Design review of the part built by this model. Coordinates are the model's own, in mm. A direction names the side the tool comes from. Coordinates: 2 decimals unless noted, no trailing zeros. Write each loop counter-clockwise with the first axis right and the second up, starting at its lowest first coordinate (ties: lowest second). Pieces come first, ordered by that corner, then holes.
Q1. Mouldability with a two-part tool opening along X and no side actions: class faces 4 (the cylindrical face through (-33.416, 29.257, 43.021)), 5 (the flat face through (35.84, 42.41, 0.21)), 6 (the cylindrical face through (4.38, -8.43, 47.54)), 7 (the flat face through (-7, -35.5, 1)) as pulls with the +X half, pulls with the -X half, needs draft (parallel to the pull), parting line crosses it, or undercut.
Q2. Take a section at A-A (z = 1.5). Give the boundary of the cut face in (x, y).
Q3. Take a section at B-B (z = -37.5). Give the boundary of the cut face in (x, y).
Q4. Machinability: for faces 1 (the flat face through (-34.09, -15.44, -42.98)), 2 (the flat face through (-33.94, 15.06, -42.98)), 3 (the flat face through (29, 40, 15)), which of the approach directions +Z, -Z, +X, -X, +Y, -Y give a long, thin tool a straight path to every point of the face, cutting with its end or side? Answer none if there is none.
Q5. Take a section at C-C (y = -16). Give the boundary of the cut face in (x, z), and give its area (3 significant figures).
Q6. For probe 1 along Y at (x, z) = (28, -1.75); probe 2 along X at (y, z) = (7.5, -36.5); probe 3 along Z at (x, y) = (-31.5, -30.5), list the stretches that pass through material, from the lowest coordinate up.
Q7. Take a section at D-D (x = 4.5). Give the boundary of the cut face in (y, z).
Q8. Insertion check: pin 1 (8 mm diameter, centred on y = 6, z = -27, fed in from +X); pin 2 (6 mm diameter, centred on x = -29.5, z = -9, fed in from -Y); pin 3 (8 mm diameter, centred on x = -34, y = 37, fed in from +Z); pin 4 (3 mm diameter, centred on x = -31.5, y = 27.5, fed in from -Z). Each pin has a flat end and moves straight along its axis. Give the tip position at first contact, or say it passes through.
```python
from build123d import *

# Parameters (mm, degrees)
SKETCH_1_W          = 46
SKETCH_1_H          = 89
EXTRUDE_1_DEPTH     = 35.5
SKETCH_3_R          = 2.6
EXTRUDE_2_DEPTH     = 3
EXTRUDE_START       = -3
SKETCH_4_R          = 2.6
EXTRUDE_3_DEPTH     = 3
SKETCH_5_R          = 14
EXTRUDE_4_DEPTH     = 6
SKETCH_6_R          = 11.5
CUT_EXTRUDE_1_DEPTH = 88.954242748
SKETCH_7_R          = 2.6
EXTRUDE_5_DEPTH     = 15
SKETCH_8_R          = 1.9
SKETCH_8_R_2        = 4.5
EXTRUDE_6_DEPTH     = 15
SKETCH_9_R          = 2.6
CUT_EXTRUDE_2_DEPTH = 115.249255194
SKETCH_10_R         = 9.5
CUT_EXTRUDE_3_DEPTH = 6
SKETCH_11_R         = 7.5
CUT_EXTRUDE_4_DEPTH = 6
SKETCH_12_R         = 9.5
CUT_EXTRUDE_5_DEPTH = 6


with BuildPart() as part:
    # 草图1 → 凸台-拉伸1 (new, symmetric)
    with BuildSketch(Plane(origin=(0, 0, 0), x_dir=(1, 0, 0), z_dir=(0, 1, 0))):
        Rectangle(SKETCH_1_W, SKETCH_1_H)
    extrude(amount=EXTRUDE_1_DEPTH, both=True)

    # 草图3 → 凸台-拉伸2 (add)
    # profile 1 of 2: a face of its own
    with BuildSketch(Plane.XY.offset(44.5)):
        with BuildLine():
            Line((23, 35.5), (34.653402281, 35.5))
            ThreePointArc((34.653402281, 35.5), (38.786905937, 33.313209471), (39.304766934, 28.66565901))
            Line((39.304766934, 28.66565901), (28.72340208, 1.83434099))
            ThreePointArc((28.72340208, 1.83434099), (28.374766733, 0), (28.72340208, -1.83434099))
            Line((28.72340208, -1.83434099), (39.304766934, -28.66565901))
            ThreePointArc((39.304766934, -28.66565901), (38.786905937, -33.313209471), (34.653402281, -35.5))
            Line((34.653402281, -35.5), (23, -35.5))
            Line((23, -35.5), (23, 35.5))
        make_face()
        with Locations((31.5, 27.5)):
            Circle(SKETCH_3_R, mode=Mode.SUBTRACT)
        with Locations((31.5, -27.5)):
            Circle(SKETCH_3_R, mode=Mode.SUBTRACT)
    # profile 2 of 2: a face of its own
    with BuildSketch(Plane.XY.offset(44.5)):
        with BuildLine():
            Line((-23, -35.5), (-23, 35.5))
            Line((-23, 35.5), (-34.653402281, 35.5))
            ThreePointArc((-34.653402281, 35.5), (-38.786905937, 33.313209471), (-39.304766934, 28.66565901))
            Line((-39.304766934, 28.66565901), (-28.72340208, 1.83434099))
            ThreePointArc((-28.72340208, 1.83434099), (-28.374766733, 0), (-28.72340208, -1.83434099))
            Line((-28.72340208, -1.83434099), (-39.304766934, -28.66565901))
            ThreePointArc((-39.304766934, -28.66565901), (-38.786905937, -33.313209471), (-34.653402281, -35.5))
            Line((-34.653402281, -35.5), (-23, -35.5))
        make_face()
        with Locations((-31.5, -27.5)):
            Circle(SKETCH_3_R, mode=Mode.SUBTRACT)
        with Locations((-31.5, 27.5)):
            Circle(SKETCH_3_R, mode=Mode.SUBTRACT)
    extrude(amount=-EXTRUDE_2_DEPTH)

    # 草图4 → 凸台-拉伸3 (add)
    # profile 1 of 2: a face of its own
    with BuildSketch(Plane(origin=(0, 0, -44.5), x_dir=(-1, 0, 0), z_dir=(0, 0, -1)).offset(EXTRUDE_START)):
        with BuildLine():
            Line((39.304766934, -28.66565901), (28.72340208, -1.83434099))
            ThreePointArc((28.72340208, -1.83434099), (28.374766733, 0), (28.72340208, 1.83434099))
            Line((28.72340208, 1.83434099), (39.304766934, 28.66565901))
            ThreePointArc((39.304766934, 28.66565901), (38.786905937, 33.313209471), (34.653402281, 35.5))
            Line((34.653402281, 35.5), (23, 35.5))
            Line((23, 35.5), (23, -35.5))
            Line((23, -35.5), (34.653402281, -35.5))
            ThreePointArc((34.653402281, -35.5), (38.786905937, -33.313209471), (39.304766934, -28.66565901))
        make_face()
        with Locations(Location((31.5, 27.5, 0), (0, 0, 180))):
            Circle(SKETCH_4_R, mode=Mode.SUBTRACT)
        with Locations(Location((31.5, -27.5, 0), (0, 0, 180))):
            Circle(SKETCH_4_R, mode=Mode.SUBTRACT)
    # profile 2 of 2: a face of its own
    with BuildSketch(Plane(origin=(0, 0, -44.5), x_dir=(-1, 0, 0), z_dir=(0, 0, -1)).offset(EXTRUDE_START)):
        with BuildLine():
            Line((-23, 35.5), (-34.653402281, 35.5))
            ThreePointArc((-34.653402281, 35.5), (-38.786905937, 33.313209471), (-39.304766934, 28.66565901))
            Line((-39.304766934, 28.66565901), (-28.72340208, 1.83434099))
            ThreePointArc((-28.72340208, 1.83434099), (-28.374766733, 0), (-28.72340208, -1.83434099))
            Line((-28.72340208, -1.83434099), (-39.304766934, -28.66565901))
            ThreePointArc((-39.304766934, -28.66565901), (-38.786905937, -33.313209471), (-34.653402281, -35.5))
            Line((-34.653402281, -35.5), (-23, -35.5))
            Line((-23, -35.5), (-23, 35.5))
        make_face()
        with Locations(Location((-31.5, -27.5, 0), (0, 0, 180))):
            Circle(SKETCH_4_R, mode=Mode.SUBTRACT)
        with Locations(Location((-31.5, 27.5, 0), (0, 0, 180))):
            Circle(SKETCH_4_R, mode=Mode.SUBTRACT)
    extrude(amount=EXTRUDE_3_DEPTH)

    # 草图5 → 凸台-拉伸4 (add)
    with BuildSketch(Plane.XY.offset(44.5)):
        Circle(SKETCH_5_R)
    extrude(amount=EXTRUDE_4_DEPTH)

    # 草图6 → 切除-拉伸1 (cut, through all)
    with BuildSketch(Plane(origin=(23, 0, 0), x_dir=(0, 0, -1), z_dir=(1, 0, 0))):
        with Locations((-1.5, 0)):
            Circle(SKETCH_6_R)
    extrude(amount=-CUT_EXTRUDE_1_DEPTH, mode=Mode.SUBTRACT)

    # 草图7 → 凸台-拉伸5 (add, symmetric)
    with BuildSketch(Plane.XY):
        with BuildLine():
            Line((23, 19.5), (23, 35.5))
            Line((23, 35.5), (31.5, 35.5))
            ThreePointArc((31.5, 35.5), (39.5, 27.5), (31.5, 19.5))
            Line((31.5, 19.5), (23, 19.5))
        make_face()
        with Locations((31.5, 27.5)):
            Circle(SKETCH_7_R, mode=Mode.SUBTRACT)
    extrude_5 = extrude(amount=EXTRUDE_5_DEPTH, both=True)

    # 镜向1: 凸台-拉伸5 across plane
    add(extrude_5.mirror(Plane(origin=(0, 0, 0), x_dir=(0, 0, 1), z_dir=(1, 0, 0))))

    # 草图8 → 凸台-拉伸6 (add, symmetric)
    # profile 1 of 2: a face of its own
    with BuildSketch(Plane.XY):
        with BuildLine():
            Line((39.235581788, 29.539797639), (32.351264755, 55.647386172))
            ThreePointArc((32.351264755, 55.647386172), (32.46266128, 55.078493129), (32.5, 54.5))
            ThreePointArc((32.5, 54.5), (28, 50), (23.5, 54.5))
            Line((23.5, 54.5), (23.5, 35.5))
            Line((23.5, 35.5), (31.5, 35.5))
            ThreePointArc((31.5, 35.5), (36.382705136, 33.837127942), (39.235581788, 29.539797639))
        make_face()
        with Locations((28, 42.5)):
            Circle(SKETCH_8_R, mode=Mode.SUBTRACT)
    # profile 2 of 2: a face of its own
    with BuildSketch(Plane.XY):
        with Locations((28, 54.5)):
            Circle(SKETCH_8_R_2)
        with Locations((28, 54.5)):
            Circle(SKETCH_8_R, mode=Mode.SUBTRACT)
    extrude_6 = extrude(amount=EXTRUDE_6_DEPTH, both=True)

    # 镜向2: 凸台-拉伸5, 凸台-拉伸6 across plane
    add(extrude_5.mirror(Plane(origin=(0, 0, 0), x_dir=(0, 0, 1), z_dir=(1, 0, 0))))
    add(extrude_6.mirror(Plane(origin=(0, 0, 0), x_dir=(0, 0, 1), z_dir=(1, 0, 0))))

    # 草图9 → 切除-拉伸2 (cut, through all)
    with BuildSketch(Plane.XZ.offset(35.5)):
        with Locations(Location((15, -37.5, 0), (0, 0, 270))):
            Circle(SKETCH_9_R)
        with Locations(Location((-15, -37.5, 0), (0, 0, 270))):
            Circle(SKETCH_9_R)
        with Locations(Location((-15, 37.5, 0), (0, 0, 270))):
            Circle(SKETCH_9_R)
        with Locations(Location((15, 37.5, 0), (0, 0, 270))):
            Circle(SKETCH_9_R)
    extrude(amount=-CUT_EXTRUDE_2_DEPTH, mode=Mode.SUBTRACT)

    # 草图10 → 切除-拉伸3 (cut)
    with BuildSketch(Plane.XY.offset(50.5)):
        Circle(SKETCH_10_R)
    extrude(amount=-CUT_EXTRUDE_3_DEPTH, mode=Mode.SUBTRACT)

    # 草图11 → 切除-拉伸4 (cut)
    with BuildSketch(Plane.XY.offset(44.5)):
        Circle(SKETCH_11_R)
    extrude(amount=-CUT_EXTRUDE_4_DEPTH, mode=Mode.SUBTRACT)

    # 草图12 → 切除-拉伸5 (cut)
    with BuildSketch(Plane.XY.offset(38.5)):
        Circle(SKETCH_12_R)
    extrude(amount=-CUT_EXTRUDE_5_DEPTH, mode=Mode.SUBTRACT)


solid = part.part
```
Response:
1. face 4: undercut
1. face 5: pulls with the +X half
1. face 6: undercut
1. face 7: needs draft
2. outline: (-39.24, 29.54) arc R8 ccw to (-31.5, 19.5) - (-23, 19.5) - (-23, 11.5) - (23, 11.5) - (23, 19.5) - (31.5, 19.5) arc R8 ccw to (39.24, 29.54) - (32.35, 55.65) arc R4.5 ccw to (23.5, 54.5) - (23.5, 35.5) - (-23.5, 35.5) - (-23.5, 54.5) arc R4.5 ccw to (-32.35, 55.65) - close; (-23, -35.5) - (23, -35.5) - (23, -11.5) - (-23, -11.5) - close; hole circle Ø5.2 at (-31.5, 27.5); hole circle Ø3.8 at (-28, 42.5); hole circle Ø3.8 at (-28, 54.5); hole circle Ø3.8 at (28, 42.5); hole circle Ø3.8 at (28, 54.5); hole circle Ø5.2 at (31.5, 27.5)
3. outline: (-23, -35.5) - (-17.6, -35.5) - (-17.6, 35.5) - (-23, 35.5) - close; (-12.4, -35.5) - (12.4, -35.5) - (12.4, 35.5) - (-12.4, 35.5) - close; (17.6, -35.5) - (23, -35.5) - (23, 35.5) - (17.6, 35.5) - close
4. face 1: +Z, -Z, -X
4. face 2: -Z, -X
4. face 3: +X, +Y, -Y
5. outline: (-34.31, -44.5) - (34.31, -44.5) - (34.31, -41.5) - (23, -41.5) - (23, 41.5) - (34.31, 41.5) - (34.31, 44.5) - (-34.31, 44.5) - (-34.31, 41.5) - (-23, 41.5) - (-23, -41.5) - (-34.31, -41.5) - close; hole circle Ø5.2 at (-15, -37.5); hole circle Ø5.2 at (-15, 37.5); hole circle Ø5.2 at (15, -37.5); hole circle Ø5.2 at (15, 37.5)
5. area: 4,140 mm2
6. probe 1: y = 19.5 to 40.6, 44.4 to 52.6, 56.4 to 59
6. probe 2: x = -23 to -17.4, -12.6 to 12.6, 17.4 to 23
6. probe 3: z = -44.5 to -41.5, 41.5 to 44.5
7. outline: (-35.5, -44.5) - (35.5, -44.5) - (35.5, 44.5) - (13.26, 44.5) - (13.26, 50.5) - (8.37, 50.5) - (8.37, 44.5) - (6, 44.5) - (6, 38.5) - (8.37, 38.5) - (8.37, 32.5) - (-8.37, 32.5) - (-8.37, 38.5) - (-6, 38.5) - (-6, 44.5) - (-8.37, 44.5) - (-8.37, 50.5) - (-13.26, 50.5) - (-13.26, 44.5) - (-35.5, 44.5) - close; hole circle Ø23 at (0, 1.5)
8. pin 1: stops at x = 23
8. pin 2: stops at y = 19.5
8. pin 3: stops at z = 44.5
8. pin 4: passes through
